Build history of the part. All positions in model axes, mm. Give positions to 0.01 mm unless a question says otherwise; leave off trailing zeros. Order: outer loops, then holes, each group sorted by start corner. A loop starts at its lowest first (then second) coordinate and runs counter-clockwise, first axis right, second up. Notation, with made-up numbers: M 79,10.5 L 102,10.5 A19 cw 102,22.5 Z; hole C -25,81 d5. An arc over 180 degrees is marked long. One line per item, written item: value. Start each with the question number.
from build123d import *

# Parameters (mm, degrees)
ESBO_O1_W                = 120
ESBO_O1_H                = 120
RESSALTO_EXTRUS_O1_DEPTH = 3
ESBO_O2_W                = 100
ESBO_O2_H                = 100
CORTE_EXTRUS_O1_DEPTH    = 161.631068924
ESBO_O5_W                = 7
ESBO_O5_H                = 5
RESSALTO_EXTRUS_O2_DEPTH = 20
ESBO_O6_R                = 1.5
CORTE_EXTRUS_O2_DEPTH    = 10
ESBO_O7_R                = 1.5
CORTE_EXTRUS_O3_DEPTH    = 162.843567384
ESBO_O8_R                = 1.5
CORTE_EXTRUS_O4_DEPTH    = 148.896743526
FILETE2_R                = 2.5
ESBO_O9_W                = 100
ESBO_O9_H                = 20
RESSALTO_EXTRUS_O3_DEPTH = 3
ESBO_O10_R               = 1.5
CORTE_EXTRUS_O5_DEPTH    = 10


with BuildPart() as part:
    # Esboço1 → Ressalto-extrusão1 (new body)
    with BuildSketch(Plane.XY):
        with Locations((53.473096186, -53.653846154)):
            Rectangle(ESBO_O1_W, ESBO_O1_H)
    extrude(amount=RESSALTO_EXTRUS_O1_DEPTH)

    # Esboço2 → Corte-extrusão1 (cut, through all)
    with BuildSketch(Plane.XY.offset(3)):
        with Locations((53.473096186, -53.653846154)):
            Rectangle(ESBO_O2_W, ESBO_O2_H)
    extrude(amount=-CORTE_EXTRUS_O1_DEPTH, mode=Mode.SUBTRACT)

    # Esboço5 → Ressalto-extrusão2 (add)
    with BuildSketch(Plane(origin=(0, 0, 0), x_dir=(-1, 0, 0), z_dir=(0, 0, -1))):
        with Locations((-49.973096186, -108.653846154)):
            Rectangle(ESBO_O5_W, ESBO_O5_H)
        with Locations((-24.473096186, -108.653846154)):
            Rectangle(ESBO_O5_W, ESBO_O5_H)
    extrude(amount=RESSALTO_EXTRUS_O2_DEPTH)

    # Esboço6 → Corte-extrusão2 (cut)
    with BuildSketch(Plane(origin=(0, 0, 0), x_dir=(-1, 0, 0), z_dir=(0, 0, -1))):
        with Locations((1.526903814, -108.653846154)):
            Circle(ESBO_O6_R)
        with Locations((1.526903814, -73.653846154)):
            Circle(ESBO_O6_R)
        with Locations((1.526903814, -53.653846154)):
            Circle(ESBO_O6_R)
        with Locations((1.526903814, -33.653846154)):
            Circle(ESBO_O6_R)
        with Locations((1.526903814, 1.346153846)):
            Circle(ESBO_O6_R)
        with Locations(Location((-108.473096186, 1.346153846, 0), (0, 0, 180))):
            Circle(ESBO_O6_R)
        with Locations(Location((-108.473096186, -33.653846154, 0), (0, 0, 180))):
            Circle(ESBO_O6_R)
        with Locations(Location((-108.473096186, -53.653846154, 0), (0, 0, 180))):
            Circle(ESBO_O6_R)
        with Locations(Location((-108.473096186, -73.653846154, 0), (0, 0, 180))):
            Circle(ESBO_O6_R)
        with Locations(Location((-108.473096186, -108.653846154, 0), (0, 0, 180))):
            Circle(ESBO_O6_R)
    extrude(amount=-CORTE_EXTRUS_O2_DEPTH, mode=Mode.SUBTRACT)

    # Esboço7 → Corte-extrusão3 (cut, through all)
    with BuildSketch(Plane(origin=(0, 0, 0), x_dir=(-1, 0, 0), z_dir=(0, 0, -1))):
        with Locations((-100.473096186, -108.653846154)):
            Circle(ESBO_O7_R)
    extrude(amount=-CORTE_EXTRUS_O3_DEPTH, mode=Mode.SUBTRACT)

    # Esboço8 → Corte-extrusão4 (cut, through all)
    with BuildSketch(Plane.ZY.offset(-20.973096186)):
        with Locations((-10, -108.653846154)):
            Circle(ESBO_O8_R)
    extrude(amount=-CORTE_EXTRUS_O4_DEPTH, mode=Mode.SUBTRACT)

    # Filete2
    filete2_edges = [part.edges().sort_by_distance(p)[0] for p in [
        (49.973096186, -106.153846154, 0),
        (49.973096186, -106.153846154, -20),
        (49.973096186, -111.153846154, -20),
        (46.473096186, -108.653846154, 0),
        (53.473096186, -108.653846154, 0),
        (49.973096186, -111.153846154, 0),
        (24.473096186, -106.153846154, -20),
        (24.473096186, -111.153846154, -20),
        (24.473096186, -106.153846154, 0),
        (27.973096186, -108.653846154, 0),
        (24.473096186, -111.153846154, 0),
        (20.973096186, -108.653846154, 0),
    ]]
    fillet(filete2_edges, radius=FILETE2_R - 0.0001)  # a hair under: the kernel refuses the full size

    # Esboço9 → Ressalto-extrusão3 (add)
    with BuildSketch(Plane(origin=(0, 0, 0), x_dir=(-1, 0, 0), z_dir=(0, 0, -1))):
        with Locations((-53.473096186, -73.653846154)):
            Rectangle(ESBO_O9_W, ESBO_O9_H)
        with Locations((-53.473096186, -33.653846154)):
            Rectangle(ESBO_O9_W, ESBO_O9_H)
    extrude(amount=-RESSALTO_EXTRUS_O3_DEPTH)

    # Esboço10 → Corte-extrusão5 (cut)
    with BuildSketch(Plane(origin=(0, 0, 0), x_dir=(-1, 0, 0), z_dir=(0, 0, -1))):
        with Locations((-33.473096186, 1.346153846)):
            Circle(ESBO_O10_R)
        with Locations((-53.473096186, 1.346153846)):
            Circle(ESBO_O10_R)
        with Locations((-73.473096186, 1.346153846)):
            Circle(ESBO_O10_R)
    extrude(amount=-CORTE_EXTRUS_O5_DEPTH, mode=Mode.SUBTRACT)


solid = part.part
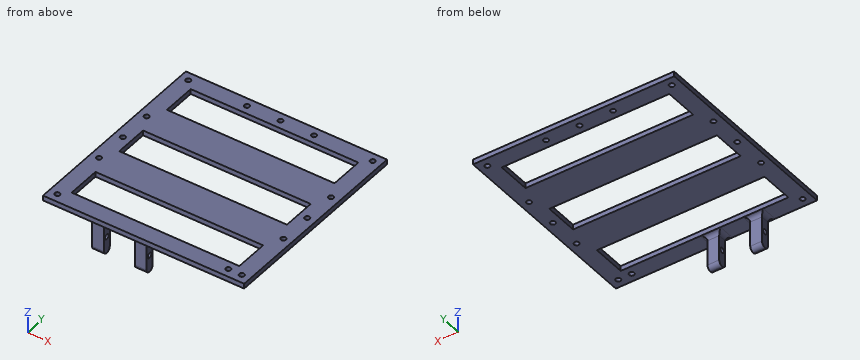
1) Slice it at A-A (x = 61.5). List the corners of the cut face in (y, z), plus the area to 3 significant figures.
2) Slice it at B-B (y = -95.5). List the corners of the cut face in (x, z), plus the area to 3 significant figures.
3) Slice it at D-D (x = 105.5). List the corners of the cut face in (y, z).
4) Drill centre lines: line 1 (Y direction, x = 26.75, z = -10); line 2 (Z direction, x = 104, y = -66); line 3 (X direction, y = -106.5, z = -12.75). Where is each one in solid material? Low to high.
5) Slice it at C-C (z = -10). List the corners of the cut face in (x, y).
6) Drop flat-ended pins along their axis: P1, Ø12, axis at x = 11.5, y = -75, coming from the -Z side; P2, Ø7.5, axis at x = 25, z = -10.5, coming from the +Y side; P3, Ø5.5, axis at x = 23.5, z = -10.5, coming from the -Y side. Give the stop position or say it passes through.
Results list:
1. outline: M -113.65,0 L -103.65,0 L -103.65,3 L -113.65,3 Z; M -83.65,0 L -63.65,0 L -63.65,3 L -83.65,3 Z; M -43.65,0 L -23.65,0 L -23.65,3 L -43.65,3 Z; M -3.65,0 L 6.35,0 L 6.35,3 L -3.65,3 Z
1. area: 180 mm²
2. outline: M -6.53,0 L 3.47,0 L 3.47,3 L -6.53,3 Z; M 103.47,0 L 113.47,0 L 113.47,3 L 103.47,3 Z
2. area: 60.0 mm²
3. outline: M -113.65,0 L 6.35,0 L 6.35,3 L -113.65,3 Z
4. line 1: y = -111.15 to -110.15, -107.15 to -106.15
4. line 2: z = 0 to 3
4. line 3: x = 20.97 to 27.97, 46.47 to 53.47
5. outline: M 20.97,-111.15 L 27.97,-111.15 L 27.97,-110.15 L 20.97,-110.15 Z; M 20.97,-107.15 L 27.97,-107.15 L 27.97,-106.15 L 20.97,-106.15 Z; M 46.47,-111.15 L 53.47,-111.15 L 53.47,-110.15 L 46.47,-110.15 Z; M 46.47,-107.15 L 53.47,-107.15 L 53.47,-106.15 L 46.47,-106.15 Z
6. P1: stops at z = 0
6. P2: stops at y = -106.15
6. P3: stops at y = -111.15
